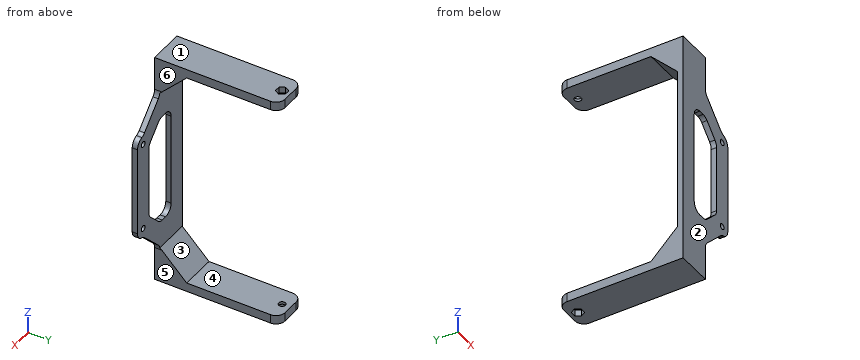
```python
from build123d import *

# Parameters (mm, degrees)
SKETCH1_W           = 20
SKETCH1_H           = 132
BOSS_EXTRUDE1_DEPTH = 3
SKETCH2_W           = 20
SKETCH2_H           = 4.999999999999993
BOSS_EXTRUDE2_DEPTH = 67
SKETCH4_R           = 1.875000000000003
CUT_EXTRUDE1_DEPTH  = 150.74645237867907
FILLET3_R           = 5
CUT_EXTRUDE2_DEPTH  = 3.5
CUT_EXTRUDE3_DEPTH  = 3.5
SKETCH9_R           = 1.625000000000004
BOSS_EXTRUDE3_DEPTH = 3
CHAMFER1_SIZE       = 15
FILLET4_R           = 5
CUT_EXTRUDE4_DEPTH  = 99.71676655968832
FILLET5_R           = 5


with BuildPart() as part:
    # Sketch1 → Boss-Extrude1 (new body)
    with BuildSketch(Plane(origin=(0, 0, 0), x_dir=(1, 0, 0), z_dir=(0, 1, 0))):
        Rectangle(SKETCH1_W, SKETCH1_H)
    extrude(amount=BOSS_EXTRUDE1_DEPTH)

    # Sketch2 → Boss-Extrude2 (add)
    with BuildSketch(Plane(origin=(0, 3, 0), x_dir=(1, 0, 0), z_dir=(0, 1, 0))):
        Polygon((-10, -66), (10, -66), (9.999999999999998, -61.00000000000001), (-10, -61.00000000000001), align=None)
        with Locations((0, 63.5)):
            Rectangle(SKETCH2_W, SKETCH2_H)
    extrude(amount=BOSS_EXTRUDE2_DEPTH)

    # Sketch4 → Cut-Extrude1 (cut, through all)
    with BuildSketch(Plane.XY.offset(66)):
        with Locations((0, 65.2375)):
            Circle(SKETCH4_R)
    extrude(amount=-CUT_EXTRUDE1_DEPTH, mode=Mode.SUBTRACT)

    # Fillet3
    fillet3_edges = [part.edges().sort_by_distance(p)[0] for p in [
        (-10, 70, 63.5),
        (10, 70, 63.5),
        (-10, 70, -63.5),
        (10, 70, -63.5),
    ]]
    fillet(fillet3_edges, radius=FILLET3_R)

    # Sketch6 → Cut-Extrude2 (cut)
    with BuildSketch(Plane.XY.offset(66)):
        Polygon((3.175426480542929, 65.2375), (1.5877132402714664, 67.9875), (-1.5877132402714669, 67.9875), (-3.1754264805429386, 65.23749999999998), (-1.5877132402714738, 62.487500000000004), (1.587713240271455, 62.487500000000004), align=None)
    extrude(amount=-CUT_EXTRUDE2_DEPTH, mode=Mode.SUBTRACT)

    # Sketch7 → Cut-Extrude3 (cut)
    with BuildSketch(Plane(origin=(0, 0, -66), x_dir=(-1, 0, 0), z_dir=(0, 0, -1))):
        Polygon((3.2042939940024326, 65.2375), (1.6021469970012208, 68.0125), (-1.6021469970012086, 68.0125), (-3.204293994002428, 65.23749999999998), (-1.6021469970012214, 62.4625), (1.602146997001218, 62.4625), align=None)
    extrude(amount=-CUT_EXTRUDE3_DEPTH, mode=Mode.SUBTRACT)

    # Sketch9 → Boss-Extrude3 (add)
    with BuildSketch(Plane.XZ):
        Polygon((30.000000000000007, -29.999999999999996), (10, -30), (10, 30.000000000000004), (30.000000000000007, 30.000000000000004), align=None)
        with Locations(Location((25, -25, 0), (0, 0, 270))):
            Circle(SKETCH9_R, mode=Mode.SUBTRACT)
        with Locations(Location((25, 25, 0), (0, 0, 270))):
            Circle(SKETCH9_R, mode=Mode.SUBTRACT)
    extrude(amount=-BOSS_EXTRUDE3_DEPTH)

    # Chamfer1
    chamfer1_edges = [part.edges().sort_by_distance(p)[0] for p in [
        (10, 1.5, 30.000000000000004),
        (10, 1.5, -30),
        (-1.78e-15, 3, 61.00000000000001),
        (0, 3, -61.00000000000001),
    ]]
    chamfer(chamfer1_edges, length=CHAMFER1_SIZE)

    # Fillet4
    fillet4_edges = [part.edges().sort_by_distance(p)[0] for p in [
        (30.000000000000007, 1.5, 30.000000000000004),
        (30.000000000000007, 1.5, -29.999999999999996),
    ]]
    fillet(fillet4_edges, radius=FILLET4_R - 0.0001)  # a hair under: the kernel refuses the full size

    # Sketch10 → Cut-Extrude4 (cut, through all)
    with BuildSketch(Plane(origin=(0, 3, 0), x_dir=(1, 0, 0), z_dir=(0, 1, 0))):
        Polygon((-7.92e-15, 30.857864376268985), (1.097e-14, -30.857864376268985), (10.00000000000001, -30.857864376268985), (20.000000000000004, -20.85786437626899), (20.000000000000004, 20.857864376268978), (9.999999999999991, 30.857864376268992), align=None)
    extrude(amount=-CUT_EXTRUDE4_DEPTH, mode=Mode.SUBTRACT)

    # Fillet5
    fillet5_edges = [part.edges().sort_by_distance(p)[0] for p in [
        (25, 1.5, 30),
        (10, 1.5, 45),
        (10, 1.5, -45),
        (25, 1.5, -29.999999999999996),
        (10.00000000000001, 1.5, 30.857864376268985),
        (1.097e-14, 1.5, 30.857864376268985),
        (-7.92e-15, 1.5, -30.857864376268985),
        (9.999999999999991, 1.5, -30.857864376268992),
        (20.000000000000004, 1.5, -20.857864376268978),
        (20.000000000000004, 1.5, 20.85786437626899),
    ]]
    fillet(fillet5_edges, radius=FILLET5_R)


solid = part.part
```
Input: part model. Units: mm. Frame: model coordinates. Face numbers are marked on the shaded views. A direction names the side the tool comes from. Give positions to 0.01 mm unless a question says otherwise; leave off trailing zeros. Order: outer loops, then holes, each group sorted by start corner. A loop starts at its lowest first (then second) coordinate and runs counter-clockwise, first axis right, second up. Notation, with made-up numbers: (32.25, -2.75) - (40.25, -2.75) arc R31 ccw to (40.25, 22.25) - close; hole circle Ø8 at (-16.5, 79.5). An arc over 180 degrees is marked (long way). One line per item, written item: value.
1. Line query: probe 1 along Z at (x, y) = (3, 18.5); probe 2 along Y at (x, z) = (0, 61.4); probe 3 along X at (y, z) = (1, 25) (3 decimals). Output: solid intervals per line, ascending.
Determined:
probe 1: -66 to -61, 61 to 66
probe 2: 0 to 63.36, 67.11 to 70
probe 3: -10 to 0, 15.858 to 23.375, 26.625 to 30
2. Reachability of the marked faces 4, 5 and 6 from +Z, -Z, +X, -X, +Y, -Y: full face, straight path, thin tool, end or side. Return the list, or none.
Determined:
face 4: +X, -X, +Y
face 5: -Z, +X, +Y, -Y
face 6: +Z, +X, +Y, -Y
3. Cut plane A-A, the plane y = 31.5. Output: boundary loops of the cut face in (x, z), and give its area (3 significant figures).
Determined:
outline: (-10, -66) - (10, -66) - (10, -61) - (-10, -61) - close; (-10, 61) - (10, 61) - (10, 66) - (-10, 66) - close
area: 200 mm2
4. Draft query along Z for the marked faces 1, 2 and 3. Return one class per face: released by +Z, released by -Z, zero draft, split by the parting line, or undercut.
Determined:
face 1: released by +Z
face 2: zero draft
face 3: undercut
5. Cut plane C-C, the plane z = -37.5. Output: boundary loops of the cut face in (x, y).
Determined:
outline: (-10, 0) - (17.5, 0) - (17.5, 3) - (-10, 3) - close
6. Cut plane B-B, the plane z = -1. Output: boundary loops of the cut face in (x, y), and give its area (3 significant figures).
Determined:
outline: (-10, 0) - (0, 0) - (0, 3) - (-10, 3) - close; (20, 0) - (30, 0) - (30, 3) - (20, 3) - close
area: 60.0 mm2
7. Pin query (flat end, axial travel): pin 1 Ø9.5 at (y, z) = (41.5, -60) entering from +X; pin 2 Ø4 at (x, z) = (13.5, -34) entering from +Y. Return the tip coordinate at first contact, or that it passes through.
Determined:
pin 1: x = 10
pin 2: y = 3
